Autodesk Inventor part; units mm, degrees
ref_plane "YZ Plane" through (0, 0, 0) normal (1, 0, 0) x (0, 1, 0)
ref_plane "XZ Plane" through (0, 0, 0) normal (0, 1, 0) x (-1, 0, 0)
ref_plane "XY Plane" through (0, 0, 0) normal (0, 0, 1) x (1, 0, 0)
sketch "Sketch2" plane through (0, 0, 0) normal (0, 1, 0) x (-1, 0, 0)
  circle A0 centre (0, 0) radius 3
  dimension "d3" = 6
extrude "Extrusion2" add sketch "Sketch2" along normal blind 11.5
sketch "Sketch3" plane through (0, 11.5, 0) normal (0, 1, 0) x (1, 0, 0)
  circle A0 centre (0, 0) radius 3
  circle A1 centre (0, 0) radius 1.5
  dimension "d6" = 3
extrude "Extrusion3" add sketch "Sketch3" along normal blind 5 contours A1
sketch "Sketch7" plane through (0, 0, 0) normal (0, -1, 0) x (1, 0, 0)
  circle A0 centre (0, 0) radius 1.5
  dimension "d16" = 3
extrude "Extrusion4" add sketch "Sketch7" along normal blind 5
sketch "Sketch8" plane through (0, -5, 0) normal (0, -1, 0) x (1, 0, 0)
  circle A0 centre (0, 0) radius 2.3
  dimension "d23" = 4.6
extrude "Extrusion5" add sketch "Sketch8" along normal blind 1
sketch "Sketch9" plane through (0, 16.5, 0) normal (0, 1, 0) x (1, 0, 0)
  circle A0 centre (0, 0) radius 2.3
  dimension "d26" = 4.6
extrude "Extrusion6" add sketch "Sketch9" along normal blind 1
fillet "Fillet2" radius 2.3 1 edges at (-2.3, 17.5, 0)
fillet "Fillet3" radius 2.3 1 edges at (-2.3, -6, 0)
properties part number "reverse gear link rod"
Work out the finished part from the listing and answer in its coordinate system (mm). A direction names the side the tool comes from. Round coordinates to 2 decimals unless told otherwise and drop trailing zeros. Write each loop counter-clockwise with the first axis right and the second up, starting at its lowest first coordinate (ties: lowest second). Pieces come first, ordered by that corner, then holes. Notation, with made-up numbers: (4.5, 79) - (17.5, 79) arc R25 ccw to (17.5, 109) - close; hole circle Ø3 at (62.25, -11). An arc over 180 degrees is marked (long way). Answer in a Markdown table with one row per item. Add a question column.
1. Given pin 1 (1.4 mm diameter, centred on x = 0.5, z = 0.5, fed in from -Y); pin 2 (1 mm diameter, centred on y = 9.5, z = 1, fed in from +X); pin 3 (1.5 mm diameter, centred on x = 1, y = 7.5, fed in from -Z); pin 4 (2 mm diameter, centred on x = 2, y = 7, fed in from +Z), each flat-ended and moving along its own axis, determine where each tip first touches the part or whether it passes through.
2. For faces 1 (the flat face through (0, -5, -2)), 2 (the flat face through (0, 17.5, 0)), determine the directions among +Z, -Z, +X, -X, +Y, -Y from which every point of the face is accessible in a straight line to the end or side of a thin tool.
3. A cutting plane is placed at B-B, the plane x = 1.85. Count the separate pieces of the cut face and the enclosed holes in it, and give its area (3 significant figures).
4. The mould has two halves that part along Y. Classify faces 3 (the flat face through (0, -6, 0)), 4 (the flat face through (0, 16.5, 2)), 5 (the cylindrical face through (-1.5, -2.46, -0.07)), 6 (the cylindrical face through (3, 6, 0)): +Y half, -Y half, draft (parallel to the pull), parting line (faces both ways), or undercut.
5. A cutting plane is placed at A-A, the plane y = 12. Determine the outline of the cut face in (x, z).
6. A cutting plane is placed at C-C, the plane y = 3.75. Determine the outline of the cut face in (x, z), and give its area (3 significant figures).
7. Find the intervals of material crossed by line 1 along Y through (x, z) = (1.55, -0.2); line 2 along Y through (x, z) = (-0.35, 2.15); line 3 along Y through (x, z) = (-2, -1.85), in increasing order. Write a range as from..to.
Worked out:
| question | item | result |
|---|---|---|
| 1 | pin 1 | y = -6 |
| 1 | pin 2 | x = 2.96 |
| 1 | pin 3 | z = -2.99 |
| 1 | pin 4 | z = 2.83 |
| 2 | face 1 | none |
| 2 | face 2 | +Z, -Z, +X, -X, +Y |
| 3 | separate pieces | 3 |
| 3 | enclosed holes | 0 |
| 3 | area | 56.2 mm^2 |
| 4 | face 3 | -Y half |
| 4 | face 4 | undercut |
| 4 | face 5 | undercut |
| 4 | face 6 | draft |
| 5 | outline | circle Ø3 at (0, 0) |
| 6 | outline | circle Ø6 at (0, 0) |
| 6 | area | 28.3 mm^2 |
| 7 | line 1 | -5.69..-5, 0..11.5, 16.5..17.19 |
| 7 | line 2 | -5.16..-5, 0..11.5, 16.5..16.66 |
| 7 | line 3 | 0..11.5 |
